```python
from build123d import *

# Parameters (mm, degrees)
SKETCH1_R           = 2.5
BOSS_EXTRUDE1_DEPTH = 3
SKETCH2_R           = 1.75
BOSS_EXTRUDE2_DEPTH = 2
SKETCH3_R           = 0.75
CUT_EXTRUDE1_DEPTH  = 6
SKETCH4_R           = 2.750200345
CUT_EXTRUDE3_DEPTH  = 4
SKETCH5_R           = 1.628426881
CUT_EXTRUDE4_DEPTH  = 0.1
FILLET1_R           = 0.3


with BuildPart() as part:
    # Sketch1 → Boss-Extrude1 (new body)
    with BuildSketch(Plane(origin=(0, 0, 0), x_dir=(1, 0, 0), z_dir=(0, 1, 0))):
        Circle(SKETCH1_R)
    extrude(amount=BOSS_EXTRUDE1_DEPTH)

    # Sketch2 → Boss-Extrude2 (add)
    with BuildSketch(Plane(origin=(0, 3, 0), x_dir=(1, 0, 0), z_dir=(0, 1, 0))):
        Circle(SKETCH2_R)
    extrude(amount=BOSS_EXTRUDE2_DEPTH)

    # Sketch3 → Cut-Extrude1 (cut, through all)
    with BuildSketch(Plane(origin=(0, 5, 0), x_dir=(1, 0, 0), z_dir=(0, 1, 0))):
        Circle(SKETCH3_R)
    extrude(amount=-CUT_EXTRUDE1_DEPTH, mode=Mode.SUBTRACT)

    # Sketch4 → Cut-Extrude3 (cut, through all)
    with BuildSketch(Plane(origin=(0, 3, 0), x_dir=(1, 0, 0), z_dir=(0, 1, 0))):
        Circle(SKETCH4_R)
        with BuildLine():
            Line((-1.71246004, 0.438726124), (-1.521118324, 0.90066589))
            Line((-1.521118324, 0.90066589), (-1.651645181, 0.954731884))
            Line((-1.651645181, 0.954731884), (-1.660451872, 0.954731884))
            ThreePointArc((-1.660451872, 0.954731884), (-1.773754473, 0.989921325), (-1.847186523, 1.083106679))
            Line((-1.847186523, 1.083106679), (-1.936085443, 1.314875773))
            ThreePointArc((-1.936085443, 1.314875773), (-1.948881988, 1.400186804), (-1.924557132, 1.482951682))
            Line((-1.924557132, 1.482951682), (-1.767766953, 1.767766953))
            Line((-1.767766953, 1.767766953), (-1.482951682, 1.924557132))
            ThreePointArc((-1.482951682, 1.924557132), (-1.400186804, 1.948881988), (-1.314875773, 1.936085443))
            Line((-1.314875773, 1.936085443), (-1.083106679, 1.847186523))
            ThreePointArc((-1.083106679, 1.847186523), (-0.989921325, 1.773754473), (-0.954731884, 1.660451872))
            Line((-0.954731884, 1.660451872), (-0.954731884, 1.651645181))
            Line((-0.954731884, 1.651645181), (-0.90066589, 1.521118324))
            Line((-0.90066589, 1.521118324), (-0.438726124, 1.71246004))
            Line((-0.438726124, 1.71246004), (-0.492792118, 1.842986897))
            Line((-0.492792118, 1.842986897), (-0.499019389, 1.849214168))
            ThreePointArc((-0.499019389, 1.849214168), (-0.554253735, 1.954213898), (-0.540286039, 2.072030195))
            Line((-0.540286039, 2.072030195), (-0.43926157, 2.298776721))
            ThreePointArc((-0.43926157, 2.298776721), (-0.387986085, 2.368149253), (-0.312262208, 2.409472589))
            Line((-0.312262208, 2.409472589), (0, 2.5))
            Line((0, 2.5), (0.312262208, 2.409472589))
            ThreePointArc((0.312262208, 2.409472589), (0.387986085, 2.368149253), (0.43926157, 2.298776721))
            Line((0.43926157, 2.298776721), (0.540286039, 2.072030195))
            ThreePointArc((0.540286039, 2.072030195), (0.554253735, 1.954213898), (0.499019389, 1.849214168))
            Line((0.499019389, 1.849214168), (0.492792118, 1.842986897))
            Line((0.492792118, 1.842986897), (0.438726124, 1.71246004))
            Line((0.438726124, 1.71246004), (0.90066589, 1.521118324))
            Line((0.90066589, 1.521118324), (0.954731884, 1.651645181))
            Line((0.954731884, 1.651645181), (0.954731884, 1.660451872))
            ThreePointArc((0.954731884, 1.660451872), (0.989921325, 1.773754473), (1.083106679, 1.847186523))
            Line((1.083106679, 1.847186523), (1.314875773, 1.936085443))
            ThreePointArc((1.314875773, 1.936085443), (1.400186804, 1.948881988), (1.482951682, 1.924557132))
            Line((1.482951682, 1.924557132), (1.767766953, 1.767766953))
            Line((1.767766953, 1.767766953), (1.924557132, 1.482951682))
            ThreePointArc((1.924557132, 1.482951682), (1.948881988, 1.400186804), (1.936085443, 1.314875773))
            Line((1.936085443, 1.314875773), (1.847186523, 1.083106679))
            ThreePointArc((1.847186523, 1.083106679), (1.773754473, 0.989921325), (1.660451872, 0.954731884))
            Line((1.660451872, 0.954731884), (1.651645181, 0.954731884))
            Line((1.651645181, 0.954731884), (1.521118324, 0.90066589))
            Line((1.521118324, 0.90066589), (1.71246004, 0.438726124))
            Line((1.71246004, 0.438726124), (1.842986897, 0.492792118))
            Line((1.842986897, 0.492792118), (1.849214168, 0.499019389))
            ThreePointArc((1.849214168, 0.499019389), (1.954213898, 0.554253735), (2.072030195, 0.540286039))
            Line((2.072030195, 0.540286039), (2.298776721, 0.43926157))
            ThreePointArc((2.298776721, 0.43926157), (2.368149253, 0.387986085), (2.409472589, 0.312262208))
            Line((2.409472589, 0.312262208), (2.5, 0))
            Line((2.5, 0), (2.409472589, -0.312262208))
            ThreePointArc((2.409472589, -0.312262208), (2.368149253, -0.387986085), (2.298776721, -0.43926157))
            Line((2.298776721, -0.43926157), (2.072030195, -0.540286039))
            ThreePointArc((2.072030195, -0.540286039), (1.954213898, -0.554253735), (1.849214168, -0.499019389))
            Line((1.849214168, -0.499019389), (1.842986897, -0.492792118))
            Line((1.842986897, -0.492792118), (1.71246004, -0.438726124))
            Line((1.71246004, -0.438726124), (1.521118324, -0.90066589))
            Line((1.521118324, -0.90066589), (1.651645181, -0.954731884))
            Line((1.651645181, -0.954731884), (1.660451872, -0.954731884))
            ThreePointArc((1.660451872, -0.954731884), (1.773754473, -0.989921325), (1.847186523, -1.083106679))
            Line((1.847186523, -1.083106679), (1.936085443, -1.314875773))
            ThreePointArc((1.936085443, -1.314875773), (1.948881988, -1.400186804), (1.924557132, -1.482951682))
            Line((1.924557132, -1.482951682), (1.767766953, -1.767766953))
            Line((1.767766953, -1.767766953), (1.482951682, -1.924557132))
            ThreePointArc((1.482951682, -1.924557132), (1.400186804, -1.948881988), (1.314875773, -1.936085443))
            Line((1.314875773, -1.936085443), (1.083106679, -1.847186523))
            ThreePointArc((1.083106679, -1.847186523), (0.989921325, -1.773754473), (0.954731884, -1.660451872))
            Line((0.954731884, -1.660451872), (0.954731884, -1.651645181))
            Line((0.954731884, -1.651645181), (0.90066589, -1.521118324))
            Line((0.90066589, -1.521118324), (0.438726124, -1.71246004))
            Line((0.438726124, -1.71246004), (0.492792118, -1.842986897))
            Line((0.492792118, -1.842986897), (0.499019389, -1.849214168))
            ThreePointArc((0.499019389, -1.849214168), (0.554253735, -1.954213898), (0.540286039, -2.072030195))
            Line((0.540286039, -2.072030195), (0.43926157, -2.298776721))
            ThreePointArc((0.43926157, -2.298776721), (0.387986085, -2.368149253), (0.312262208, -2.409472589))
            Line((0.312262208, -2.409472589), (0, -2.5))
            Line((0, -2.5), (-0.312262208, -2.409472589))
            ThreePointArc((-0.312262208, -2.409472589), (-0.387986085, -2.368149253), (-0.43926157, -2.298776721))
            Line((-0.43926157, -2.298776721), (-0.540286039, -2.072030195))
            ThreePointArc((-0.540286039, -2.072030195), (-0.554253735, -1.954213898), (-0.499019389, -1.849214168))
            Line((-0.499019389, -1.849214168), (-0.492792118, -1.842986897))
            Line((-0.492792118, -1.842986897), (-0.438726124, -1.71246004))
            Line((-0.438726124, -1.71246004), (-0.90066589, -1.521118324))
            Line((-0.90066589, -1.521118324), (-0.954731884, -1.651645181))
            Line((-0.954731884, -1.651645181), (-0.954731884, -1.660451872))
            ThreePointArc((-0.954731884, -1.660451872), (-0.989921325, -1.773754473), (-1.083106679, -1.847186523))
            Line((-1.083106679, -1.847186523), (-1.314875773, -1.936085443))
            ThreePointArc((-1.314875773, -1.936085443), (-1.400186804, -1.948881988), (-1.482951682, -1.924557132))
            Line((-1.482951682, -1.924557132), (-1.767766953, -1.767766953))
            Line((-1.767766953, -1.767766953), (-1.924557132, -1.482951682))
            ThreePointArc((-1.924557132, -1.482951682), (-1.948881988, -1.400186804), (-1.936085443, -1.314875773))
            Line((-1.936085443, -1.314875773), (-1.847186523, -1.083106679))
            ThreePointArc((-1.847186523, -1.083106679), (-1.773754473, -0.989921325), (-1.660451872, -0.954731884))
            Line((-1.660451872, -0.954731884), (-1.651645181, -0.954731884))
            Line((-1.651645181, -0.954731884), (-1.521118324, -0.90066589))
            Line((-1.521118324, -0.90066589), (-1.71246004, -0.438726124))
            Line((-1.71246004, -0.438726124), (-1.842986897, -0.492792118))
            Line((-1.842986897, -0.492792118), (-1.849214168, -0.499019389))
            ThreePointArc((-1.849214168, -0.499019389), (-1.954213898, -0.554253735), (-2.072030195, -0.540286039))
            Line((-2.072030195, -0.540286039), (-2.298776721, -0.43926157))
            ThreePointArc((-2.298776721, -0.43926157), (-2.368149253, -0.387986085), (-2.409472589, -0.312262208))
            Line((-2.409472589, -0.312262208), (-2.5, 0))
            Line((-2.5, 0), (-2.409472589, 0.312262208))
            ThreePointArc((-2.409472589, 0.312262208), (-2.368149253, 0.387986085), (-2.298776721, 0.43926157))
            Line((-2.298776721, 0.43926157), (-2.072030195, 0.540286039))
            ThreePointArc((-2.072030195, 0.540286039), (-1.954213898, 0.554253735), (-1.849214168, 0.499019389))
            Line((-1.849214168, 0.499019389), (-1.842986897, 0.492792118))
            Line((-1.842986897, 0.492792118), (-1.71246004, 0.438726124))
        make_face(mode=Mode.SUBTRACT)
    extrude(amount=-CUT_EXTRUDE3_DEPTH, mode=Mode.SUBTRACT)

    # Sketch5 → Cut-Extrude4 (cut)
    with BuildSketch(Plane.XZ):
        Circle(SKETCH5_R)
    extrude(amount=-CUT_EXTRUDE4_DEPTH, mode=Mode.SUBTRACT)

    # Fillet1
    fillet1_edges = [part.edges().sort_by_distance(p)[0] for p in [
        (-1.75, 5, 0),
    ]]
    fillet(fillet1_edges, radius=FILLET1_R)


solid = part.part
```
Check sheet for the modelled part. Datum: model origin and axes. Units: mm. A direction names the side the tool comes from. Round coordinates to 2 decimals unless told otherwise and drop trailing zeros. Loops run counter-clockwise (first coordinate to the right, second up) from the corner with the lowest first, then second, coordinate; pieces in that order, holes last. Notation, with made-up numbers: M 40.25,41.5 L 86.25,41.5 A35 ccw 86.25,75.5 Z; hole C -34,66 d4. An arc over 180 degrees is marked long. Answer as a JSON object with one key per item and string values.
1. Gauge pin test, flat ends, axial feed: P1, Ø3, axis at y = 3.5, z = -1.5, coming from the +X side; P2, Ø2.5, axis at x = -0.5, z = 0, coming from the -Y side; P3, Ø0.6, axis at x = 1.5, z = 1, coming from the +Y side. Record the tip position at first contact, or that the pin passes through.
Reply:
{"P1": "stops at x = 2.48", "P2": "stops at y = 0", "P3": "stops at y = 5"}
2. Section check B-B (z = -2.2). Record the boundary of the cut face in (x, y), plus the area to 3 significant figures.
Reply:
{"outline": "M -0.48,0 L 0.48,0 L 0.48,3 L -0.48,3 Z", "area": "2.90 mm²"}
3. Scan lines: line 1 (Z direction, x = 0, y = 3.25); line 2 (Y direction, x = -1.2, z = -0.5); line 3 (X direction, y = 2.7, z = -2). Record each from-to range of solid material in increasing order.
Reply:
{"line 1": "z = -1.75 to -0.75, 0.75 to 1.75", "line 2": "y = 0.1 to 5", "line 3": "x = -0.56 to 0.56"}
4. Section check A-A (y = 3.85). Record the boundary of the cut face in (x, z).
Reply:
{"outline": "C 0,0 d3.5; hole C 0,0 d1.5"}
5. Mould release check, pull along X, two halves, no side actions. Record for faces 1 (the flat face through (1, 0.1, 0)), 2 (the cylindrical face through (1.617, 3.838, 0.67)), 3 (the flat face through (1.4, 3, 1.4)), 4 (the cylindrical face through (-0.75, 2.58, -0.03)): pulls with the +X half, pulls with the -X half, needs draft (parallel to the pull), parting line crosses it, or undercut.
Reply:
{"face 1": "undercut", "face 2": "parting line crosses it", "face 3": "needs draft", "face 4": "undercut"}
6. Access from +Z, -Z, +X, -X, +Y, -Y to the whole of each face (thin tool, end or side, straight path). Record for faces 5 (the flat face through (1.4, 3, -1.5)), 6 (the flat face through (-1.5, 3, -1.5)), 7 (the flat face through (0, 5, 1)), 8 (the flat face through (-1.5, 3, 1.4)), 9 (the flat face through (0, 0, -2)).
Reply:
{"face 5": "-Z, +X, +Y", "face 6": "-Z, -X, +Y", "face 7": "+Z, -Z, +X, -X, +Y", "face 8": "+Z, -X, +Y", "face 9": "+Z, -Z, +X, -X, -Y"}
